Job drawing, mm, ordinate dimensions from the low corner. One solid piece. Round coordinates to 2 decimals unless told otherwise and drop trailing zeros. Write each loop counter-clockwise with the first axis right and the second up, starting at its lowest first coordinate (ties: lowest second). Pieces come first, ordered by that corner, then holes.
1) Drill centre lines: L1, parallel to X at y = 4.5, z = 5.45; L2, parallel to Y at x = 178.5, z = 5.3; L3, parallel to Y at x = 82, z = 3.1. Where is each one in solid material? Low to high.
2) Flat gauge pins, fed straight in: pin 1 (1.8 mm diameter, centred on x = 115.5, z = 2.5, fed in from +Y); pin 2 (1.8 mm diameter, centred on x = 48.5, z = 3, fed in from -Y); pin 3 (3 mm diameter, centred on y = 5.5, z = 3.5, fed in from -X). Where does each tip first touch, or does it go through?
3) Saw through at A-A on x = 195. Write the cut outline in (y, z).
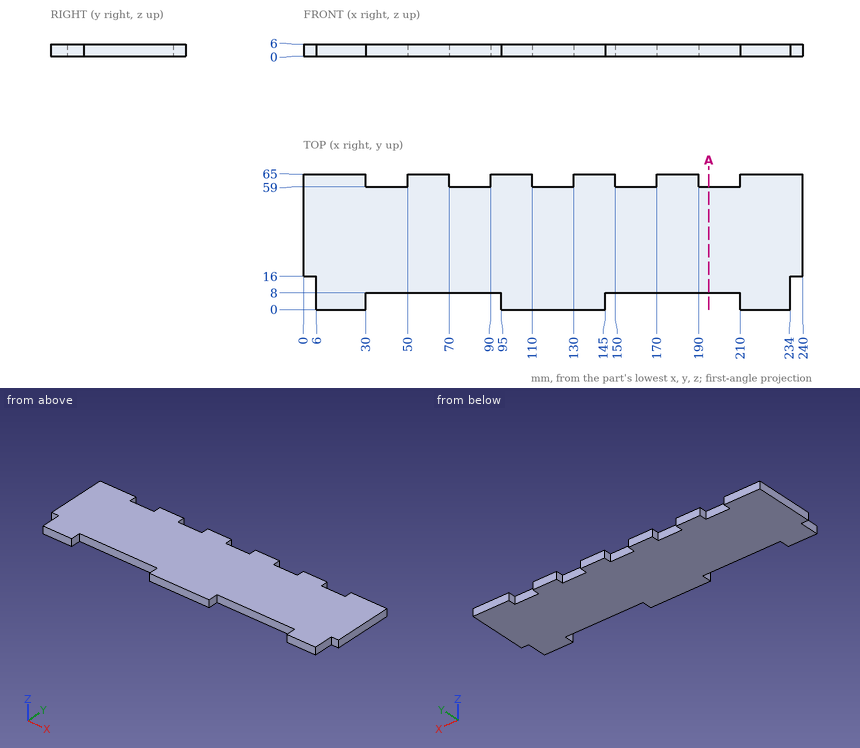
Completed:
1. L1: x = 6 to 30, 95 to 145, 210 to 234
1. L2: y = 8 to 65
1. L3: y = 8 to 59
2. pin 1: stops at y = 59
2. pin 2: stops at y = 8
2. pin 3: stops at x = 6
3. outline: (8, 0) - (59, 0) - (59, 6) - (8, 6) - close
